Autodesk Inventor part; units mm, degrees
ref_plane "YZ Plane" through (0, 0, 0) normal (1, 0, 0) x (0, 1, 0)
ref_plane "XZ Plane" through (0, 0, 0) normal (0, 1, 0) x (-1, 0, 0)
ref_plane "XY Plane" through (0, 0, 0) normal (0, 0, 1) x (1, 0, 0)
sketch "Sketch6" plane through (0, 0, 0) normal (0, 1, 0) x (-1, 0, 0)
  line L0 (0, 0) -> (22, 0)
  line L1 (22, 0) -> (22, -22)
  line L2 (22, -22) -> (0, -22)
  line L3 (0, -22) -> (0, 0)
  dimension "d18" = 22
  dimension "d19" = 22
extrude "Extrusion3" add sketch "Sketch6" along normal blind 50
ref_plane "Work Plane1" through (-11, 0, -22) normal (-1, 0, 0) x (0, 0, 1)
sketch "Sketch8" plane through (-11, 0, -22) normal (-1, 0, 0) x (0, 0, 1)
  line L0 (0, 50) -> (22, 50)
  line L1 (11, 50) -> (11, 58)
  circle A0 centre (11, 58) radius 9
  line L2 (11.0985, 49.0005) -> (10.9015, 66.9995)
  point P0 (22, 0)
  dimension "d30" = 8
  dimension "d31" = 18
revolve "Revolution2" add sketch "Sketch8" angle 360 about axis through (-11, 49.0005, -10.9015) along (0, 0.9999401, -0.0109435) picked at (12.4036, 52.6667) picked at (13.3498, 49.8198) contours A0 L0 L2 | L2 L0 A0
properties part number "queen"
Can you work these out from the model? Positions are in its coordinate system, mm. Give positions to 0.01 mm unless a question says otherwise; leave off trailing zeros. Loops run counter-clockwise (first coordinate to the right, second up) from the corner with the lowest first, then second, coordinate; pieces in that order, holes last. Notation, with made-up numbers: M -1,-38 L 46,-38 A16 cw 46,-19 Z; hole C 11,28 d6. An arc over 180 degrees is marked long. Answer in a Markdown table with one row per item.
1. Suppose I cut it at B-B on x = -15. Write out the boundary of the cut face in (y, z), plus the area to 3 significant figures.
Taken from the geometry:
| item | result |
|---|---|
| outline | M 0,-22 L 50,-22 L 50,-12 A8.06 ccw long 50,-10 L 50,0 L 0,0 Z |
| area | 1,300 mm² |
2. Suppose I cut it at C-C on x = -18.75. Write out the boundary of the cut face in (y, z), plus the area to 3 significant figures.
Taken from the geometry:
| item | result |
|---|---|
| outline | M 0,-22 L 50,-22 L 50,0 L 0,0 Z; C 58,-11 d9.15 |
| area | 1,170 mm² |
3. Thinking about a two-plate mould opening in Y: for faces 1 (the flat face through (-16, 50, -11)), 2 (the flat face through (-11, 0, -11)), 3 (the flat face through (-22, 25, -11)), which applies, released by +Y, released by -Y, zero draft, split by the parting line, or undercut?
Taken from the geometry:
| item | result |
|---|---|
| face 1 | undercut |
| face 2 | released by -Y |
| face 3 | zero draft |
4. If I drill on line 1 along Y through (x, z) = (-14.75, -1); line 2 along Y through (x, z) = (-5, -12.5); line 3 along Y through (x, z) = (-5.5, -8.25), over which ranges is the centre line in solid material (lowest first)?
Taken from the geometry:
| item | result |
|---|---|
| line 1 | y = 0 to 50 |
| line 2 | y = 0 to 50, 51.46 to 64.54 |
| line 3 | y = 0 to 50, 51.43 to 64.57 |
5. Suppose I cut it at D-D on z = -12.5. Write out the boundary of the cut face in (x, y).
Taken from the geometry:
| item | result |
|---|---|
| outline | M -22,0 L 0,0 L 0,50 L -7.16,50 A8.87 ccw long -14.84,50 L -22,50 Z |
6. For pin 1 Ø6.5 at (x, z) = (-10.5, -15.5) entering from +Y; pin 2 Ø1 at (y, z) = (59, -7.5) entering from -X, each with a flat end and sliding along its axis, tell me the tip position at first contact or that it passes through.
Taken from the geometry:
| item | result |
|---|---|
| pin 1 | stops at y = 66.91 |
| pin 2 | stops at x = -19.43 |
7. Suppose I cut it at A-A on z = -5.5. Write out the boundary of the cut face in (x, y), plus the area to 3 significant figures.
Taken from the geometry:
| item | result |
|---|---|
| outline | M -22,0 L 0,0 L 0,50 L -22,50 Z; C -11,58 d14.25 |
| area | 1,260 mm² |
